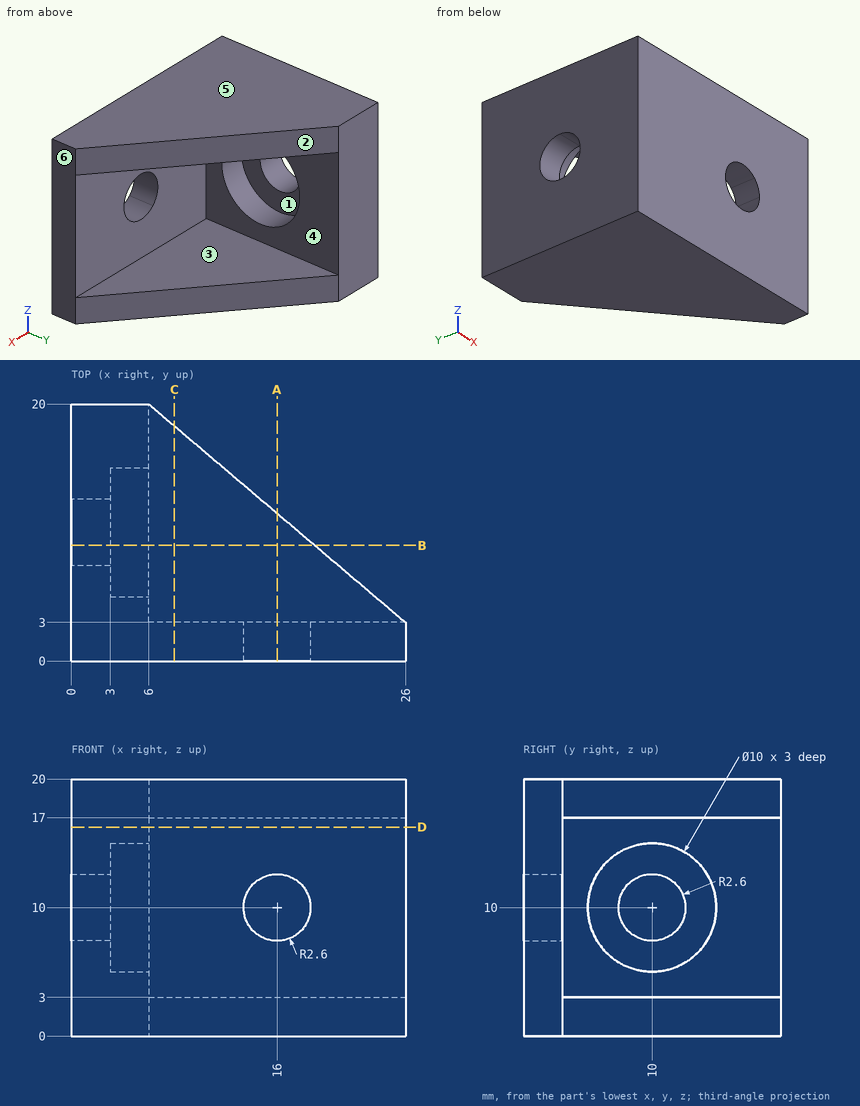
Study the drawing (mm; zero at the part's minimum x, y, z) and answer. A direction names the side the tool comes from. Coordinates: 2 decimals unless noted, no trailing zeros. Loops run counter-clockwise (first coordinate to the right, second up) from the corner with the lowest first, then second, coordinate; pieces in that order, holes last. Notation, with made-up numbers: M 19,-31.5 L 48,-31.5 A27 ccw 48,-9.5 Z; hole C 79.25,46 d9. An arc over 180 degrees is marked long. Answer in a Markdown table with one row per item. Add a question column.
1. Find section D-D, the plane z = 16.25. Write down the section's boundary in (x, y), then the cut area to 3 significant figures.
2. A tool of negligible diameter and unlimited length cuts with its end or side. For the marked faces 1, 2 and 3, from which of +Z, -Z, +X, -X, +Y, -Y can it reach the whole face along a straight path? Write none if from no direction.
3. Flat-ended cylindrical pins translate along their axes: P1, Ø8, axis at y = 17, z = 8.5, coming from the +X side; P2, Ø5, axis at y = 8, z = 9.5, coming from the +X side; P3, Ø1.5, axis at y = 4.5, z = 3.5, coming from the +X side. Find the tip coordinate at first contact, or state that the pin passes through.
4. Find section B-B, the plane y = 9. Write down the section's boundary in (x, z).
5. The mould has two halves that part along Z. Classify the marked faces 4, 5 and 6: pulls with the +Z half, pulls with the -Z half, needs draft (parallel to the pull), parting line crosses it, or undercut.
6. Consider L1, parallel to Y at x = 4.25, z = 10; L2, parallel to Z at x = 6.5, y = 17.5. Determine where each line is inside the solid, lowest interval first.
7. Find section A-A, the plane x = 16. Write down the section's boundary in (y, z).
8. Find section C-C, the plane x = 8. Write down the section's boundary in (y, z), then the cut area to 3 significant figures.
Reported:
| question | item | result |
|---|---|---|
| 1 | outline | M 0,0 L 26,0 L 26,3 L 6,3 L 6,20 L 0,20 Z |
| 1 | area | 180 mm^2 |
| 2 | face 1 | +X |
| 2 | face 2 | +Z, -Z, +X, +Y |
| 2 | face 3 | +X, +Y |
| 3 | P1 | stops at x = 6 |
| 3 | P2 | stops at x = 3 |
| 3 | P3 | stops at x = 24.89 |
| 4 | outline | M 0,0 L 18.94,0 L 18.94,3 L 6,3 L 6,5.1 L 3,5.1 L 3,7.6 L 0,7.6 Z; M 0,12.4 L 3,12.4 L 3,14.9 L 6,14.9 L 6,17 L 18.94,17 L 18.94,20 L 0,20 Z |
| 5 | face 4 | undercut |
| 5 | face 5 | pulls with the +Z half |
| 5 | face 6 | needs draft |
| 6 | L1 | y = 0 to 5, 15 to 20 |
| 6 | L2 | z = 0 to 3, 17 to 20 |
| 7 | outline | M 0,0 L 11.5,0 L 11.5,3 L 3,3 L 3,7.4 L 0,7.4 Z; M 0,12.6 L 3,12.6 L 3,17 L 11.5,17 L 11.5,20 L 0,20 Z |
| 8 | outline | M 0,0 L 18.3,0 L 18.3,3 L 3,3 L 3,17 L 18.3,17 L 18.3,20 L 0,20 Z |
| 8 | area | 152 mm^2 |
